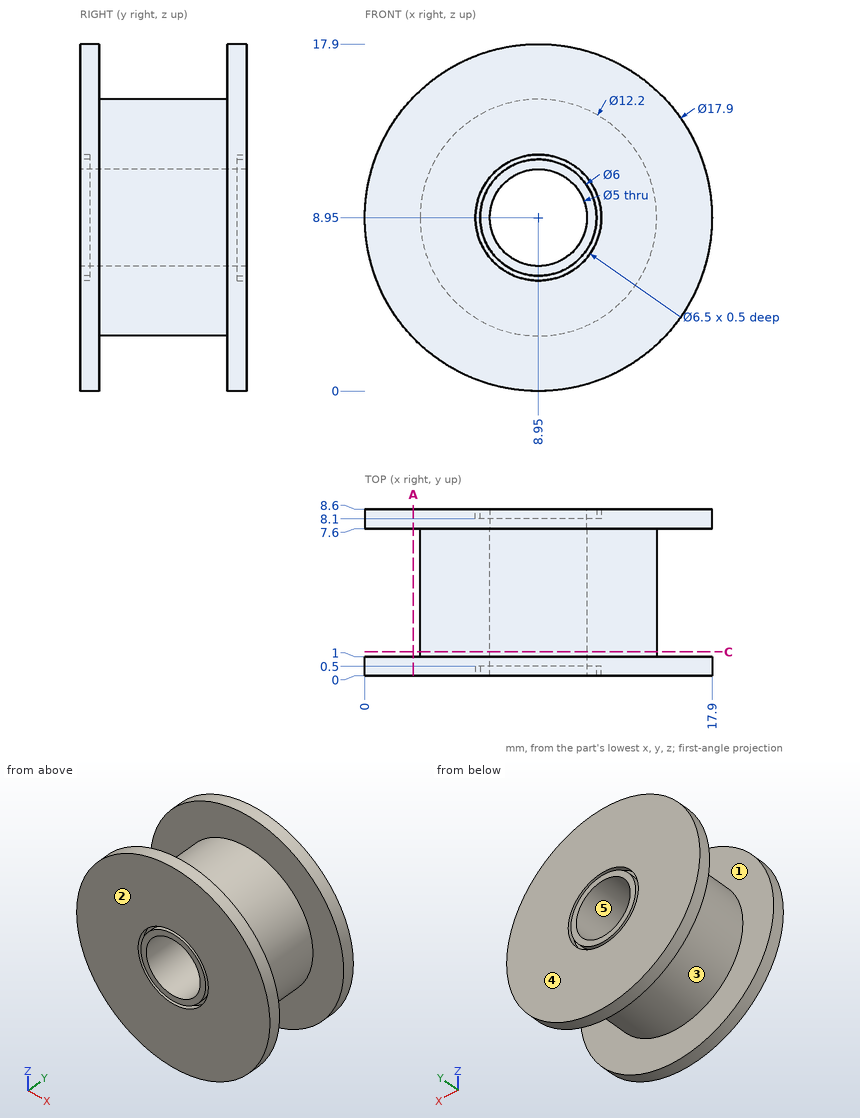
Drawing for the job (mm, zero at the part's lowest x, y, z). A direction names the side the tool comes from. Give positions to 0.01 mm unless a question says otherwise; leave off trailing zeros. Order: outer loops, then holes, each group sorted by start corner. A loop starts at its lowest first (then second) coordinate and runs counter-clockwise, first axis right, second up. Notation, with made-up numbers: M 14,81.25 L 31,81.25 A18 cw 31,109.25 Z; hole C 20,66 d3. An arc over 180 degrees is marked long. Write item = value, one per line. Start each with the question number.
(1) Which spindle directions (+Z, -Z, +X, -X, +Y, -Y) get a long thin tool onto all of the face, cutting with end or side? Do the marked faces 1 and 2. Say none if no direction does.
(2) Slice it at A-A on x = 2.5. Write the cut outline in (y, z), plus the area to 3 significant figures.
(3) Two-plate mould, pull along X, no slides. Class the marked faces 3, 4 and 5: released by +X, released by -X, zero draft, split by the parting line, or undercut.
(4) Slice it at C-C on y = 1.25. Write the cut outline in (x, z), plus the area to 3 significant figures.
(5) Probe L1, parallel to Z at x = 8.95, y = 8.5; L2, parallel to Z at x = 8.95, y = 6. List the from-to ranges inside material, lowest first. Write a range as [from, to].
(6) Pin check, flat tips, straight feed: pin 1 Ø5 at (x, z) = (2, 11.5) entering from -Y; pin 2 Ø1 at (x, y) = (15, 5.5) entering from -Z; pin 3 Ø1 at (y, z) = (3.5, 9) entering from -X; pin 4 Ø1.5 at (y, z) = (6, 5) entering from -X. Stop position of each tip, or through.
Responses:
q1.face_1 = none
q1.face_2 = +Z, -Z, +X, -X, -Y
q2.outline = M 0,2.75 L 1,2.75 L 1,15.15 L 0,15.15 Z; M 7.6,2.75 L 8.6,2.75 L 8.6,15.15 L 7.6,15.15 Z
q2.area = 24.8 mm2
q3.face_3 = split by the parting line
q3.face_4 = zero draft
q3.face_5 = undercut
q4.outline = C 8.95,8.95 d12.2; hole C 8.95,8.95 d5
q4.area = 97.3 mm2
q5.L1 = [0, 5.7], [5.95, 6.45], [11.45, 11.95], [12.2, 17.9]
q5.L2 = [2.85, 6.45], [11.45, 15.05]
q6.pin_1 = 0
q6.pin_2 = 6.42
q6.pin_3 = 2.85
q6.pin_4 = 3.76
